Input: part model. Units: mm. Frame: model coordinates. Face numbers are marked on the shaded views. A direction names the side the tool comes from. Round coordinates to 2 decimals unless told otherwise and drop trailing zeros. Write each loop counter-clockwise with the first axis right and the second up, starting at its lowest first coordinate (ties: lowest second). Pieces come first, ordered by that corner, then holes. Notation, with made-up numbers: (62.5, -17.5) -> (91.5, -17.5) arc R18 cw to (91.5, 7.5) -> close; hole circle Ø11 at (-24.75, 10). An arc over 180 degrees is marked (long way). Write item = value, one per line.
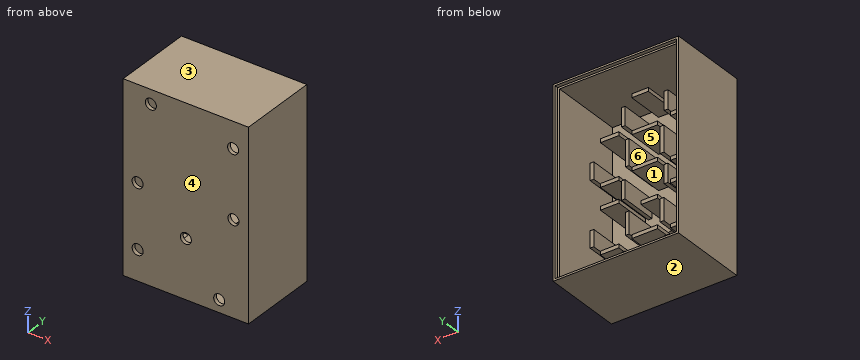
```python
from build123d import *

# Parameters (mm, degrees)
SKETCH287_W     = 68
SKETCH287_H     = 102
PAD198_DEPTH    = 43.5
SKETCH288_W     = 64
SKETCH288_H     = 98
POCKET042_DEPTH = 41.5
SKETCH289_W     = 66
SKETCH289_H     = 100
POCKET043_DEPTH = 2
SKETCH290_W     = 2
SKETCH290_H     = 9
SKETCH290_H_2   = 12
SKETCH290_H_3   = 14
SKETCH290_H_4   = 10
SKETCH290_W_2   = 10
SKETCH290_H_5   = 2
PAD199_DEPTH    = 20
SKETCH291_R     = 3
POCKET044_DEPTH = 5


with BuildPart() as part:
    # Sketch287 → Pad198 (new body)
    with BuildSketch(Plane.XZ):
        Rectangle(SKETCH287_W, SKETCH287_H)
    extrude(amount=-PAD198_DEPTH)

    # Sketch288 (on Face6 of Pad198) → Pocket042 (cut)
    with BuildSketch(Plane(origin=(0, 43.5, 0), x_dir=(1, 0, 0), z_dir=(0, 1, 0))):
        Rectangle(SKETCH288_W, SKETCH288_H)
    extrude(amount=-POCKET042_DEPTH, mode=Mode.SUBTRACT)

    # Sketch289 (on Face5 of Pocket042) → Pocket043 (cut)
    with BuildSketch(Plane(origin=(0, 43.5, 0), x_dir=(1, 0, 0), z_dir=(0, 1, 0))):
        Rectangle(SKETCH289_W, SKETCH289_H)
    extrude(amount=-POCKET043_DEPTH, mode=Mode.SUBTRACT)

    # Sketch290 (on Face16 of Pocket043) → Pad199 (join)
    with BuildSketch(Plane(origin=(0, 2, 0), x_dir=(1, 0, 0), z_dir=(0, 1, 0))):
        with Locations((28.6, 20)):
            Rectangle(SKETCH290_W, SKETCH290_H)
        with Locations((28.6, -15)):
            Rectangle(SKETCH290_W, SKETCH290_H)
        with Locations((9.4, 19)):
            Rectangle(SKETCH290_W, SKETCH290_H_2)
        with Locations((9.4, -17.5)):
            Rectangle(SKETCH290_W, SKETCH290_H_3)
        with Locations((11.6, 1)):
            Rectangle(SKETCH290_W, SKETCH290_H_4)
        with Locations((11.6, 38)):
            Rectangle(SKETCH290_W, SKETCH290_H_4)
        Polygon((0, 47.1), (2, 47.1), (2, 45.1), (0, 45.1), (-7, 45.1), (-7, 47.1), align=None)
        Polygon((0, 27.9), (7, 27.9), (7, 25.9), (0, 25.9), (-7, 25.9), (-7, 27.9), align=None)
        Polygon((0, 12.1), (2, 12.1), (2, 10.1), (0, 10.1), (-7, 10.1), (-7, 12.1), align=None)
        Polygon((0, -7.1), (7, -7.1), (7, -9.1), (0, -9.1), (-7, -9.1), (-7, -7.1), align=None)
        Polygon((0, -25.9), (7, -25.9), (7, -27.9), (0, -27.9), (-7, -27.9), (-7, -25.9), align=None)
        with Locations((11.6, -37)):
            Rectangle(SKETCH290_W, SKETCH290_H_4)
        Polygon((0, -45.1), (7, -45.1), (7, -47.1), (0, -47.1), (-2, -47.1), (-2, -45.1), align=None)
        with Locations((19, 5.9)):
            Rectangle(SKETCH290_W_2, SKETCH290_H_5)
        with Locations((19, -5.9)):
            Rectangle(SKETCH290_W_2, SKETCH290_H_5)
        with Locations((19, -29.1)):
            Rectangle(SKETCH290_W_2, SKETCH290_H_5)
        with Locations((19, 29.1)):
            Rectangle(SKETCH290_W_2, SKETCH290_H_5)
        with Locations((-28.6, 15)):
            Rectangle(SKETCH290_W, SKETCH290_H)
        with Locations((-28.6, -20)):
            Rectangle(SKETCH290_W, SKETCH290_H)
        with Locations((-9.4, 19)):
            Rectangle(SKETCH290_W, SKETCH290_H_2)
        with Locations((-9.4, -17.5)):
            Rectangle(SKETCH290_W, SKETCH290_H_3)
        with Locations((-11.6, 1)):
            Rectangle(SKETCH290_W, SKETCH290_H_4)
        with Locations((-11.6, 38)):
            Rectangle(SKETCH290_W, SKETCH290_H_4)
        with Locations((-11.6, -37)):
            Rectangle(SKETCH290_W, SKETCH290_H_4)
        with Locations((-19, 5.9)):
            Rectangle(SKETCH290_W_2, SKETCH290_H_5)
        with Locations((-19, -5.9)):
            Rectangle(SKETCH290_W_2, SKETCH290_H_5)
        with Locations((-19, -29.1)):
            Rectangle(SKETCH290_W_2, SKETCH290_H_5)
        with Locations((-19, 29.1)):
            Rectangle(SKETCH290_W_2, SKETCH290_H_5)
    extrude(amount=PAD199_DEPTH)

    # Sketch291 (on Face16 of Pad199) → Pocket044 (cut)
    with BuildSketch(Plane(origin=(0, 2, 0), x_dir=(1, 0, 0), z_dir=(0, 1, 0))):
        with Locations((-26.14077, 34.68518)):
            Circle(SKETCH291_R)
        with Locations((18.10867, 44.321499)):
            Circle(SKETCH291_R)
        with Locations((25.819803, 0)):
            Circle(SKETCH291_R)
        with Locations((25.639233, -36.743561)):
            Circle(SKETCH291_R)
        with Locations((-18.966691, -43.366471)):
            Circle(SKETCH291_R)
        with Locations((-26.180906, 0)):
            Circle(SKETCH291_R)
        with Locations((0, 19.229425)):
            Circle(SKETCH291_R)
    extrude(amount=-POCKET044_DEPTH, mode=Mode.SUBTRACT)


with BuildPart() as part_1:
    # Body062 placement: moved
    add(part.part.moved(Location((0, -31.5, 0))))


solid = part_1.part
```
1) Cut plane D-D (y = -14.5). Count the separate pieces of the cut face and the enclosed holes in it, and give its area (3 significant figures).
Solutions:
separate_pieces = 29
enclosed_holes = 1
area = 1,260 mm^2
2) Cut plane C-C (z = 22.5). Return the cut outline in (x, y).
Solutions:
outline = (-34, -31.5) -> (34, -31.5) -> (34, 12) -> (33, 12) -> (33, 10) -> (32, 10) -> (32, -29.5) -> (10.4, -29.5) -> (10.4, -9.5) -> (8.4, -9.5) -> (8.4, -29.5) -> (-8.4, -29.5) -> (-8.4, -9.5) -> (-10.4, -9.5) -> (-10.4, -29.5) -> (-27.6, -29.5) -> (-27.6, -9.5) -> (-29.6, -9.5) -> (-29.6, -29.5) -> (-32, -29.5) -> (-32, 10) -> (-33, 10) -> (-33, 12) -> (-34, 12) -> close
3) Access query for the marked faces 1 and 2. Directions: +Z, -Z, +X, -X, +Y, -Y. A direction counts if a zero-diameter tool reaches every point of the face in a straight line with its end or side. Return the directions, or none.
Solutions:
face_1 = +Y
face_2 = -Z, +X, -X, +Y, -Y
4) Cut plane B-B (y = 8). Return the cut outline in (x, z), and give its area (3 significant figures).
Solutions:
outline = (-34, -51) -> (34, -51) -> (34, 51) -> (-34, 51) -> close; hole (-32, -49) -> (32, -49) -> (32, 49) -> (-32, 49) -> close
area = 664 mm^2
5) Draft query along Z for the marked faces 3, 4, 5 and 6. Return one class per face: +Z half, -Z half, draft (parallel to the pull), parting line (faces both ways), or undercut.
Solutions:
face_3 = +Z half
face_4 = draft
face_5 = undercut
face_6 = undercut
6) First-contact query: P1, Ø5, axis at x = 25.64, z = 36.74, coming from the -Y side; P2, Ø2, axis at x = -19.5, z = -6, coming from the +Y side. Flat tips, straight axial feed; report the tip coordinate or a pass-through.
Solutions:
P1 = through
P2 = -9.5
7) Cut plane A-A (z = 0). Return the cut outline in (x, y).
Solutions:
outline = (-34, -31.5) -> (-29.18, -31.5) -> (-29.18, -29.5) -> (-32, -29.5) -> (-32, 10) -> (-33, 10) -> (-33, 12) -> (-34, 12) -> close; (-23.18, -31.5) -> (22.82, -31.5) -> (22.82, -29.5) -> (12.6, -29.5) -> (12.6, -9.5) -> (10.6, -9.5) -> (10.6, -29.5) -> (-10.6, -29.5) -> (-10.6, -9.5) -> (-12.6, -9.5) -> (-12.6, -29.5) -> (-23.18, -29.5) -> close; (28.82, -31.5) -> (34, -31.5) -> (34, 12) -> (33, 12) -> (33, 10) -> (32, 10) -> (32, -29.5) -> (28.82, -29.5) -> close
8) Line query: L1, parallel to X at y = -16.5, z = 32.5; L2, parallel to Z at x = 3, y = -10.5; L3, parallel to Z at x = -20, y = -10. Output: solid intervals per line, ascending. Write a range as from..to.
Solutions:
L1 = -34..-32, -12.6..-10.6, 10.6..12.6, 32..34
L2 = -51..-49, -27.9..-25.9, 7.1..9.1, 25.9..27.9, 45.1..47.1, 49..51
L3 = -51..-49, -30.1..-28.1, -6.9..-4.9, 4.9..6.9, 28.1..30.1, 49..51
